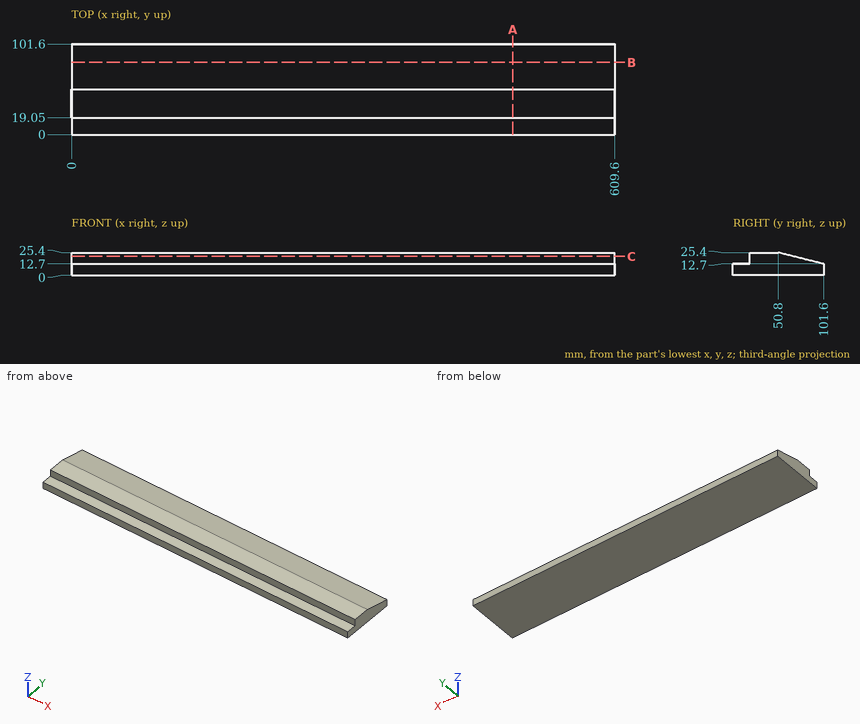
Geometry: see drawing. Coordinates: mm, zero at the bounding-box minimum. Give positions to 0.01 mm unless a question says otherwise; leave off trailing zeros. Loops run counter-clockwise (first coordinate to the right, second up) from the corner with the lowest first, then second, coordinate; pieces in that order, holes last. Notation, with made-up numbers: M 8,58 L 56,58 A5 ccw 56,66 Z; hole C 24.5,-24.75 d10. An arc over 180 degrees is marked long. Answer as CSV lines item,"result". Start each with the question number.
1. Pin query (flat end, axial travel): P1, Ø4, axis at x = 156.5, y = 88.5, coming from the +Z side (3 decimals); P2, Ø5.5, axis at x = 421.5, y = 8.5, coming from the +Z side; P3, Ø3, axis at y = 26, z = 13.5, coming from the -X side. Return the tip coordinate at first contact, or that it passes through.
2. Line query: L1, parallel to Z at x = 384.5, y = 19; L2, parallel to Z at x = 222, y = 62. Output: solid intervals per line, ascending.
3. Section B-B on y = 81. Return loops of the section in (x, z).
4. Section A-A on x = 495. Return loops of the section in (y, z), plus the area to 3 significant figures.
5. Section C-C on z = 21.25. Return loops of the section in (x, y).
Computed values:
1,P1,"stops at z = 16.475"
1,P2,"stops at z = 12.7"
1,P3,"stops at x = 0"
2,L1,"z = 0 to 12.7"
2,L2,"z = 0 to 22.6"
3,outline,"M 0,0 L 609.6,0 L 609.6,17.85 L 0,17.85 Z"
4,outline,"M 0,0 L 101.6,0 L 101.6,12.7 L 50.8,25.4 L 19.05,25.4 L 19.05,12.7 L 0,12.7 Z"
4,area,"2,020 mm²"
5,outline,"M 0,19.05 L 609.6,19.05 L 609.6,67.4 L 0,67.4 Z"
